Design review of the part shown in the three views and the two pictorial views. Dimensions are in mm from the part's minimum x, y and z. A direction names the side the tool comes from. Round coordinates to 2 decimals unless told otherwise and drop trailing zeros. Order: outer loops, then holes, each group sorted by start corner. A loop starts at its lowest first (then second) coordinate and runs counter-clockwise, first axis right, second up. Notation, with made-up numbers: (-3.75, -13.75) -> (38.25, -13.75) arc R16 ccw to (38.25, 14.25) -> close; hole circle Ø1 at (66, 87). An arc over 180 degrees is marked (long way). Put each result on its own line as item: value. Start each with the question number.
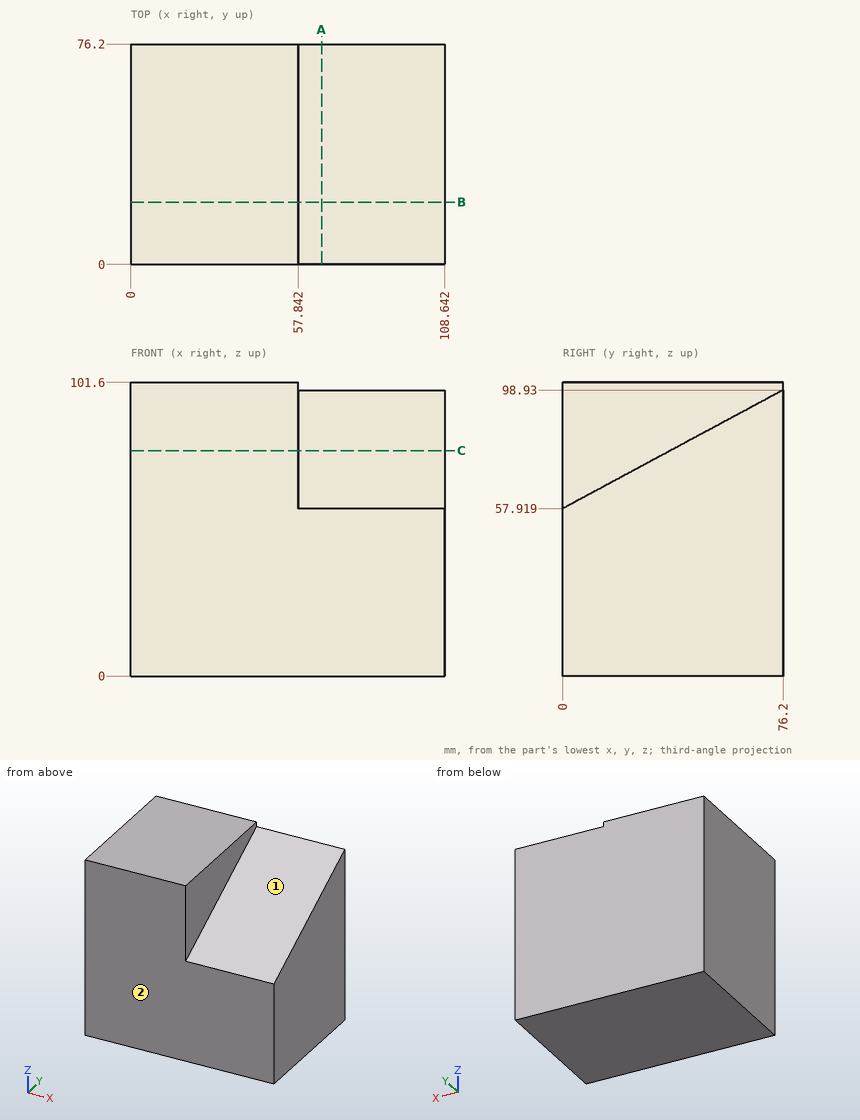
Q1. Take a section at A-A on x = 66. Give the boundary of the cut face in (y, z).
Q2. Clearance check with flat-ended pins moving along their axes: pin 1 Ø1.5 at (x, y) = (92, 18.5) entering from +Z; pin 2 Ø6 at (x, y) = (65, 16.5) entering from +Z. State where each tip first meets the part, or that it passes through.
Q3. Take a section at C-C on z = 78. Give the boundary of the cut face in (x, y).
Q4. Take a section at B-B on y = 21.5. Give the boundary of the cut face in (x, z), and give its area (3 significant figures).
Q5. For the marked faces 1 and 2, list the 3-axis set-ups (+Z, -Z, +X, -X, +Y, -Y) from which the entire face can be reached by the end or side of a thin tool; tool diameter is ignored.
Q6. Wall thickness on probe 1 along X at (y, z) = (35, 84.5); probe 2 along Z at (x, y) = (91, 64) (1 decimal); probe 3 along Z at (x, y) = (64, 64.5): over which ranges is each line inside the solid? List them lowest first. Write a range as [from, to].
Calculated:
1. outline: (0, 0) -> (76.2, 0) -> (76.2, 98.93) -> (0, 57.92) -> close
2. pin 1: stops at z = 68.28
2. pin 2: stops at z = 68.41
3. outline: (0, 0) -> (57.84, 0) -> (57.84, 37.31) -> (108.64, 37.31) -> (108.64, 76.2) -> (0, 76.2) -> close
4. outline: (0, 0) -> (108.64, 0) -> (108.64, 69.49) -> (57.84, 69.49) -> (57.84, 101.6) -> (0, 101.6) -> close
4. area: 9,410 mm²
5. face 1: +Z, +X, -Y
5. face 2: +Z, -Z, +X, -X, -Y
6. probe 1: x = [0, 57.84]
6. probe 2: z = [0, 92.4]
6. probe 3: z = [0, 92.63]
